from build123d import *

# Parameters (mm, degrees)
BOSS_EXTRUDE1_DEPTH = 6
CUT_EXTRUDE1_DEPTH  = 6
SKETCH3_W           = 6
SKETCH3_H           = 6
BOSS_EXTRUDE2_DEPTH = 8
SKETCH5_W           = 8
SKETCH5_H           = 3.1
CUT_EXTRUDE2_DEPTH  = 8
SKETCH6_R           = 0.975
CUT_EXTRUDE3_DEPTH  = 8
SKETCH7_W           = 6
SKETCH7_H           = 3
BOSS_EXTRUDE3_DEPTH = 8
SKETCH8_R           = 1.025
CUT_EXTRUDE4_DEPTH  = 8
FILLET1_R           = 3
FILLET2_R           = 1


with BuildPart() as part:
    # Sketch1 → Boss-Extrude1 (new body)
    with BuildSketch(Plane(origin=(0, 0, 0), x_dir=(1, 0, 0), z_dir=(0, 1, 0))):
        with BuildLine():
            ThreePointArc((59.197580629, 1.463473077), (28.251548273, 20.077561964), (-2.65465833, 1.397422323))
            ThreePointArc((-2.65465833, 1.397422323), (-1.397422323, -2.65465833), (2.65465833, -1.397422323))
            ThreePointArc((2.65465833, -1.397422323), (28.257955548, 14.077565385), (53.894245187, -1.342704605))
            ThreePointArc((53.894245187, -1.342704605), (57.949001749, -2.591283485), (59.197580629, 1.463473077))
        make_face()
    extrude(amount=BOSS_EXTRUDE1_DEPTH)

    # Sketch2 → Cut-Extrude1 (cut)
    with BuildSketch(Plane(origin=(0, 6, 0), x_dir=(1, 0, 0), z_dir=(0, 1, 0))):
        Polygon((53.894245187, -1.342704605), (59.197580629, 1.463473077), (61.240293877, -2.397007189), (55.867953369, -5.072773667), align=None)
        Polygon((2.65465833, -1.397422323), (-2.65465833, 1.397422323), (-5.113209947, -2.397007189), (1.520441913, -5.715494495), align=None)
    extrude(amount=-CUT_EXTRUDE1_DEPTH, mode=Mode.SUBTRACT)

    # Sketch3 → Boss-Extrude2 (add)
    with BuildSketch(Plane(origin=(12.343879945, 0, 23.328435834), x_dir=(0.883889240381717, 0, -0.46769628044002154), z_dir=(0.4676962804400216, 0, 0.8838892403817171))):
        with Locations((50.008565489, 3)):
            Rectangle(SKETCH3_W, SKETCH3_H)
    extrude(amount=BOSS_EXTRUDE2_DEPTH)

    # Sketch5 → Cut-Extrude2 (cut)
    with BuildSketch(Plane(origin=(46.853700684, 0, -24.791908911), x_dir=(-0.46769628044002165, 0, -0.883889240381717), z_dir=(0.883889240381717, 0, -0.46769628044002165))):
        with Locations((-30.392940165, 3)):
            Rectangle(SKETCH5_W, SKETCH5_H)
    extrude(amount=-CUT_EXTRUDE2_DEPTH, mode=Mode.SUBTRACT)

    # Sketch6 → Cut-Extrude3 (cut)
    with BuildSketch(Plane(origin=(0, 6, 0), x_dir=(1, 0, 0), z_dir=(0, 1, 0))):
        with Locations(Location((58.88439431, -4.359061966, 0), (0, 0, 270))):
            Circle(SKETCH6_R)
    extrude(amount=-CUT_EXTRUDE3_DEPTH, mode=Mode.SUBTRACT)

    # Sketch7 → Boss-Extrude3 (add)
    with BuildSketch(Plane(origin=(0, 0, 0), x_dir=(0.8848861101120022, 0, 0.4658074410428085), z_dir=(-0.4658074410428085, 0, 0.8848861101120022))):
        with Locations((0, 3)):
            Rectangle(SKETCH7_W, SKETCH7_H)
    extrude(amount=BOSS_EXTRUDE3_DEPTH)

    # Sketch8 → Cut-Extrude4 (cut)
    with BuildSketch(Plane(origin=(0, 4.5, 0), x_dir=(1, 0, 0), z_dir=(0, 1, 0))):
        with Locations(Location((-2.329037205, -4.424430551, 0), (0, 0, 180))):
            Circle(SKETCH8_R)
    extrude(amount=-CUT_EXTRUDE4_DEPTH, mode=Mode.SUBTRACT)

    # Fillet1
    fillet1_edges = [part.edges().sort_by_distance(p)[0] for p in [
        (57.63581543, 5.275, 8.413818528),
        (57.63581543, 0.725, 8.413818528),
        (62.939150873, 0.725, 5.607640846),
        (62.939150873, 5.275, 5.607640846),
        (-1.071801198, 3, 8.476511204),
        (-6.381117859, 3, 5.681666558),
    ]]
    fillet(fillet1_edges, radius=FILLET1_R - 0.0001)  # a hair under: the kernel refuses the full size

    # Fillet2
    fillet2_edges = [part.edges().sort_by_distance(p)[0] for p in [
        (28.251548273, 0, -20.077561964),
        (28.251548273, 6, -20.077561964),
        (60.366844715, 0, 0.746294218),
        (61.751579759, 0, 5.241952749),
        (58.001503527, 0, 7.226247414),
        (55.063509273, 0, 3.552471901),
        (60.366844715, 6, 0.746294218),
        (61.751579759, 6, 5.241952749),
        (58.001503527, 6, 7.226247414),
        (55.063509273, 6, 3.552471901),
        (53.894245187, 3, 1.342704605),
        (59.197580629, 3, -1.463473077),
        (0, 0, 0),
        (0, 6, 0),
        (28.257955548, 0, -14.077565385),
        (28.257955548, 6, -14.077565385),
    ]]
    fillet(fillet2_edges, radius=FILLET2_R)


solid = part.part
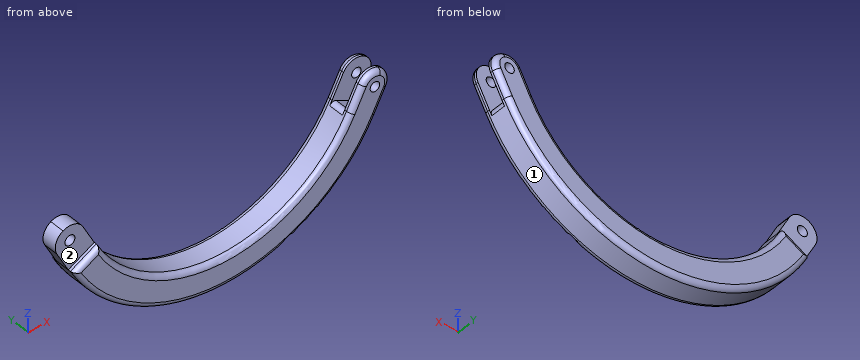
Can you work these out from the model? Positions are in its coordinate system, mm. Face numbers are marked on the shaded views. A direction names the side the tool comes from. Give positions to 0.01 mm unless a question says otherwise; leave off trailing zeros. Answer in a Markdown table with one row per item. Add a question column.
Item 1: On a 3-axis mill with a long thin cutter (end or side, diameter ignored), from which of +Z, -Z, +X, -X, +Y, -Y can I reach the whole of each face in a straight line? I mean the marked faces 1 and 2. Say none if no direction works.
Item 2: For pin 1 Ø6.5 at (x, z) = (-2.5, 3.5) entering from +Y; pin 2 Ø3 at (x, y) = (2, 1.5) entering from +Z; pin 3 Ø2.5 at (x, z) = (-0.5, 4) entering from -Y, each with a flat end and sliding along its axis, tell me the tip position at first contact or that it passes through.
Item 3: Please list where these lines run through material, in increasing order: L1, parallel to X at y = 1.25, z = 1.25; L2, parallel to X at y = 1, z = -3.25; L3, parallel to Z at x = 58, y = 1.
Evaluation:
| question | item | result |
|---|---|---|
| 1 | face 1 | -Z, +Y, -Y |
| 1 | face 2 | +Z, -X, -Y |
| 2 | pin 1 | stops at y = 4.5 |
| 2 | pin 2 | stops at z = 5.49 |
| 2 | pin 3 | stops at y = 1.5 |
| 3 | L1 | x = 2.37 to 2.73, 53.84 to 60.63 |
| 3 | L2 | x = -1.61 to 5.7, 50.87 to 58.18 |
| 3 | L3 | z = -3.55 to 3.95, 4.77 to 7.23 |
